Build history of the part. All positions in model axes, mm. A direction names the side the tool comes from. Give positions to 0.01 mm unless a question says otherwise; leave off trailing zeros. Loops run counter-clockwise (first coordinate to the right, second up) from the corner with the lowest first, then second, coordinate; pieces in that order, holes last. Notation, with made-up numbers: (23.5, -17.75) - (82.5, -17.75) arc R30 ccw to (82.5, 14.25) - close; hole circle Ø8 at (1.5, 35). An arc over 180 degrees is marked (long way). Return JSON: item names as keys, results as strings. Group by question number.
1) Drop flat-ended pins along their axis: pin 1 (1.5 mm diameter, centred on y = 7.5, z = 9.5, fed in from +X); pin 2 (5 mm diameter, centred on x = 45, z = 13, fed in from +Y); pin 3 (3 mm diameter, centred on x = 23.5, y = 4, fed in from +Z); pin 4 (6 mm diameter, centred on x = 17.5, y = 7.5, fed in from -Z). Give the stop position or say it passes through.
2) Slice it at A-A (x = 23). List the corners of the cut face in (y, z).
3) Slice it at C-C (x = 1). List the corners of the cut face in (y, z).
4) Mould opens along Z. For faces 4 (the face through (22.86, 9.699, 4.715)), 5 (the face through (23, 10, 3)), 6 (the face through (24.526, -1.521, 11.481)) say: released by +Z, released by -Z, zero draft, split by the parting line, or undercut.
5) Slice it at B-B (y = -1). List the corners of the cut face in (x, z).
6) Slice it at D-D (y = 2.25). List the corners of the cut face in (x, z), and give its area (3 significant figures).
7) 3-axis set-ups, long thin cutter, end or side, ignore diameter. For faces 1 (the face through (39, 5, 10)), 2 (the face through (0, 5, 5)), 3 (the face through (22.9, 3.6, 5)): which of +Z, -Z, +X, -X, +Y, -Y reach the whole face in a straight line?
8) Drill centre lines: probe 1 along Z at (x, y) = (23, -0.6); probe 2 along X at (y, z) = (2.25, 6.75); probe 3 along Y at (x, z) = (43, 4.5). Where is each one in solid material? Low to high. Write a range as from..to.
Autodesk Inventor part; units mm, degrees
ref_plane "YZ Plane" through (0, 0, 0) normal (1, 0, 0) x (0, 1, 0)
ref_plane "XZ Plane" through (0, 0, 0) normal (0, 1, 0) x (-1, 0, 0)
ref_plane "XY Plane" through (0, 0, 0) normal (0, 0, 1) x (1, 0, 0)
sketch "Sketch1" plane through (0, 0, 0) normal (0, 0, 1) x (1, 0, 0)
  line L0 (0, 0) -> (46, 0)
  line L1 (46, 0) -> (46, 10)
  line L2 (46, 10) -> (0, 10)
  line L3 (0, 10) -> (0, 0)
  circle A0 centre (3, 7) radius 1.5
  circle A1 centre (43, 7) radius 1.5
  circle A2 centre (13, 3) radius 3
  circle A3 centre (33, 3) radius 3
  line L4 (18, 7) -> (28, 7)
  line L5 (28, 7) -> (28, 4)
  line L6 (28, 4) -> (18, 4)
  line L7 (18, 4) -> (18, 7)
  point P0 (23, 7)
  point P1 (23, 10)
  dimension "d2" = 10
  dimension "d3" = 3
  dimension "d4" = 3
  dimension "d5" = 3
  dimension "d6" = 3
  dimension "d7" = 3
  dimension "d8" = 40
  dimension "d11" = 6
  dimension "d12" = 6
  dimension "d13" = 10
  dimension "d14" = 10
  dimension "d26" = 7
  dimension "d27" = 10
  dimension "d28" = 3
extrude "Extrusion1" add sketch "Sketch1" along normal blind 10 contours A2 | A3 | L3 L2 L1 L0
sketch "Sketch2" plane through (0, 0, 10) normal (0, 0, 1) x (1, 0, 0)
  line L0 (46, 10) -> (0, 10)
  line L1 (0, 0) -> (46, 0)
  line L2 (13, 10) -> (33, 10)
  line L3 (33, 10) -> (33, 0)
  line L4 (33, 0) -> (13, 0)
  line L5 (13, 0) -> (13, 10)
  point P0 (23, 10)
  point P1 (23, 10)
  dimension "d15" = 20
extrude "Extrusion2" cut sketch "Sketch2" against normal blind 5
sketch "Sketch3" plane through (0, 0, 0) normal (0, -1, 0) x (1, 0, 0)
  line L0 (-2, 16) -> (48, 16)
  line L1 (48, 16) -> (48, 0)
  line L2 (48, 0) -> (-2, 0)
  line L3 (-2, 0) -> (-2, 16)
  line L4 (0, 10) -> (13, 10)
  line L5 (0, 0) -> (0, 10)
  line L6 (46, 0) -> (46, 10)
  line L7 (0, 0) -> (46, 0)
  point P0 (23, 16)
  point P1 (23, 0)
  dimension "d19" = 6
  dimension "d22" = 0
  dimension "d30" = 50
extrude "Extrusion3" add sketch "Sketch3" along normal blind 3
fillet "Fillet1" radius 1 4 edges at (23, 10, 5) (23, 10, 0) (23, 7, 0) (23, 7, 5)
sketch "Sketch4" plane through (0, -3, 0) normal (0, -1, 0) x (1, 0, 0)
  circle A0 centre (1, 13) radius 1.6
  circle A1 centre (45, 13) radius 1.6
  line L0 (48, 16) -> (-2, 16)
  circle A2 centre (23, 11) radius 1.6
  point P0 (0, 0)
  point P1 (23, 16)
  dimension "d32" = 3.2
  dimension "d33" = 3.2
  dimension "d34" = 3
  dimension "d35" = 3
  dimension "d36" = 3
  dimension "d37" = 3
  dimension "d38" = 3.2
  dimension "d39" = 5
extrude "Extrusion4" cut sketch "Sketch4" against normal blind 10
equation "\"d11\" = d12"
equation "\"d19\" = d20"
equation "\"d32\" = d38"
equation "\"d33\" = d38"
properties part number "z endcap"
Results:
{
 "1": {"pin 1": "x = 46", "pin 2": "y = 0", "pin 3": "z = 5", "pin 4": "z = 0"},
 "2": {"outline": "(-3, 0) - (4, 0) - (4, 5) - (0, 5) - (0, 9.4) - (-3, 9.4) - close; (-3, 12.6) - (0, 12.6) - (0, 16) - (-3, 16) - close; (7, 1) arc R1 ccw to (8, 0) - (9, 0) arc R1 ccw to (10, 1) - (10, 4) arc R1 ccw to (9, 5) - (8, 5) arc R1 ccw to (7, 4) - close"},
 "3": {"outline": "(-3, 0) - (9, 0) arc R1 ccw to (10, 1) - (10, 10) - (0, 10) - (0, 11.4) - (-3, 11.4) - close; (-3, 14.6) - (0, 14.6) - (0, 16) - (-3, 16) - close"},
 "4": {"face 4": "released by +Z", "face 5": "zero draft", "face 6": "undercut"},
 "5": {"outline": "(-2, 0) - (48, 0) - (48, 16) - (-2, 16) - close; hole circle Ø3.2 at (1, 13); hole circle Ø3.2 at (23, 11); hole circle Ø3.2 at (45, 13)"},
 "6": {"outline": "(0, 0) - (46, 0) - (46, 10) - (33, 10) - (33, 5) - (13, 5) - (13, 10) - (0, 10) - close", "area": "360 mm2"},
 "7": {"face 1": "+Z, +X, -X, +Y", "face 2": "+Z, -Z, -X, +Y", "face 3": "+Z, +Y"},
 "8": {"probe 1": "0..9.4, 12.6..16", "probe 2": "0..13, 33..46", "probe 3": "-3..5.5, 8.5..10"}
}
